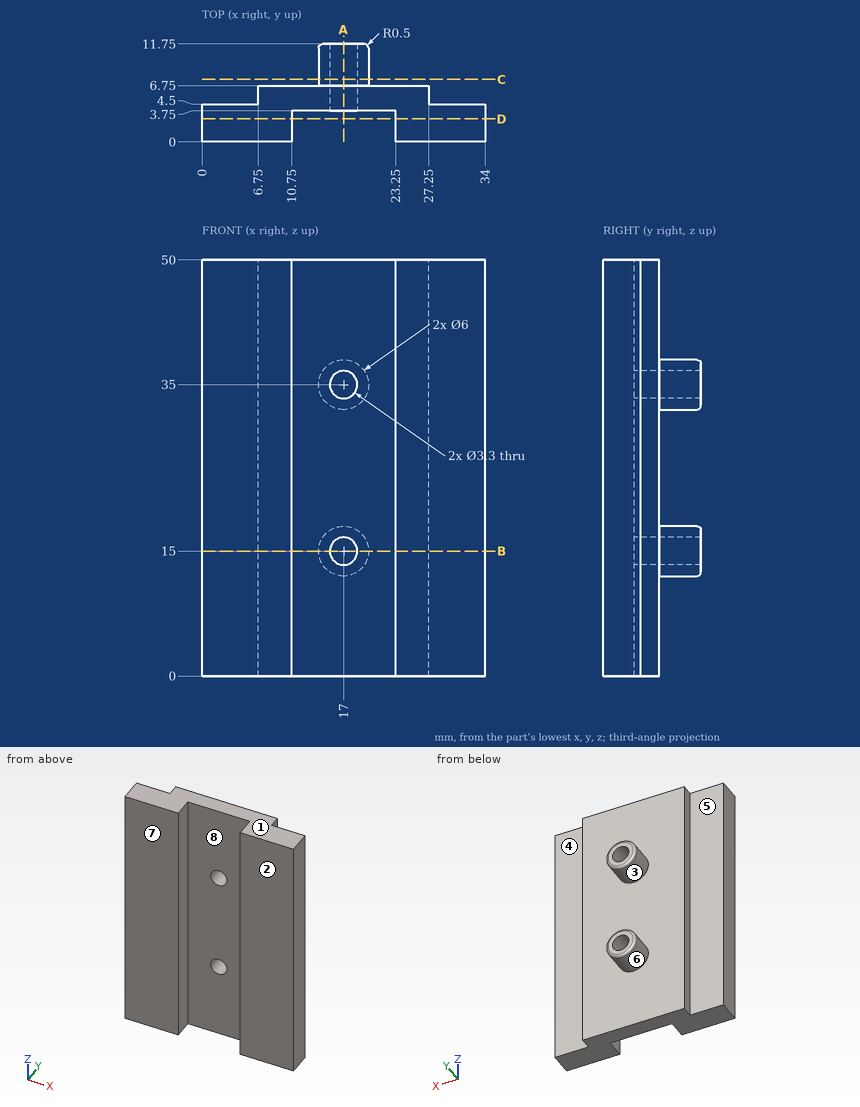
The figure shows three views and two pictorial views of one solid part (mm, origin at its lowest corner). Answer the questions. A direction names the side the tool comes from. Give positions to 0.01 mm unless a question says otherwise; leave off trailing zeros. Write each loop counter-clockwise with the first axis right and the second up, starting at its lowest first coordinate (ties: lowest second). Pieces come first, ordered by that corner, then holes. Notation, with made-up numbers: M 2,66 L 39,66 A15 ccw 39,81 Z; hole C 52,78.5 d8. An arc over 180 degrees is marked long. One line per item, written item: value. Start each with the question number.
(1) Find the intervals of material crossed by line 1 (X direction, y = 1.5, z = 35); line 2 (X direction, y = 6, z = 35); line 3 (Y direction, x = 7, z = 17), in increasing order.
(2) Find section B-B (z = 15). Determine the outline of the cut face in (x, y), plus the area to 3 significant figures.
(3) Flat-ended cylindrical pins translate along their axes: pin 1 Ø1.5 at (x, y) = (23, 2.5) entering from +Z; pin 2 Ø6 at (x, z) = (17, 25) entering from -Y; pin 3 Ø3 at (y, z) = (6.5, 33.5) entering from -X; pin 4 Ø2 at (y, z) = (7.5, 26.5) entering from +X. Find the tip coordinate at first contact, or state that the pin passes through.
(4) Find section C-C (y = 7.5). Determine the outline of the cut face in (x, z), plus the area to 3 significant figures.
(5) A tool of negligible diameter and unlimited length cuts with its end or side. For the marked faces 1, 2, 3, 4 and 5, from which of +Z, -Z, +X, -X, +Y, -Y can it reach the whole face along a straight path? Write none if from no direction.
(6) Determine the mould class of the marked faces 6, 7 and 8 for opening direction X: pulls with the +X half, pulls with the -X half, needs draft (parallel to the pull), parting line crosses it, or undercut.
(7) Find section D-D (y = 2.75). Determine the outline of the cut face in (x, z), plus the area to 4 significant figures.
(8) Find section A-A (x = 17). Determine the outline of the cut face in (y, z).
Results below:
1. line 1: x = 0 to 10.75, 23.25 to 34
1. line 2: x = 6.75 to 15.35, 18.65 to 27.25
1. line 3: y = 0 to 6.75
2. outline: M 0,0 L 10.75,0 L 10.75,3.75 L 15.35,3.75 L 15.35,11.75 L 14.5,11.75 A0.5 ccw 14,11.25 L 14,6.75 L 6.75,6.75 L 6.75,4.5 L 0,4.5 Z; M 18.65,3.75 L 23.25,3.75 L 23.25,0 L 34,0 L 34,4.5 L 27.25,4.5 L 27.25,6.75 L 20,6.75 L 20,11.25 A0.5 ccw 19.5,11.75 L 18.65,11.75 Z
2. area: 156 mm^2
3. pin 1: stops at z = 50
3. pin 2: stops at y = 3.75
3. pin 3: stops at x = 6.75
3. pin 4: stops at x = 27.25
4. outline: C 17,15 d6; C 17,35 d6; hole C 17,15 d3.3; hole C 17,35 d3.3
4. area: 39.4 mm^2
5. face 1: +Z, +X, -X, +Y, -Y
5. face 2: +Z, -Z, +X, -X, -Y
5. face 3: +Y
5. face 4: +Z, -Z, +X, +Y
5. face 5: +Z, -Z, -X, +Y
6. face 6: parting line crosses it
6. face 7: needs draft
6. face 8: undercut
7. outline: M 0,0 L 10.75,0 L 10.75,50 L 0,50 Z; M 23.25,0 L 34,0 L 34,50 L 23.25,50 Z
7. area: 1,075 mm^2
8. outline: M 3.75,0 L 6.75,0 L 6.75,12 L 11.25,12 A0.5 ccw 11.75,12.5 L 11.75,13.35 L 3.75,13.35 Z; M 3.75,16.65 L 11.75,16.65 L 11.75,17.5 A0.5 ccw 11.25,18 L 6.75,18 L 6.75,32 L 11.25,32 A0.5 ccw 11.75,32.5 L 11.75,33.35 L 3.75,33.35 Z; M 3.75,36.65 L 11.75,36.65 L 11.75,37.5 A0.5 ccw 11.25,38 L 6.75,38 L 6.75,50 L 3.75,50 Z
